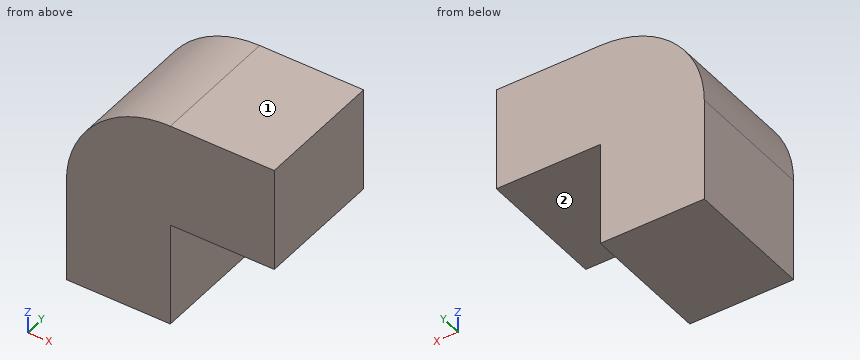
from build123d import *

# Parameters (mm, degrees)
SKETCH_1_W      = 4
SKETCH_1_H      = 5
EXTRUDE_1_DEPTH = 8
SKETCH_2_W      = 4
SKETCH_2_H      = 5
EXTRUDE_2_DEPTH = 4
FILLET_2_R      = 4


with BuildPart() as part:
    # 草图1 → 凸台-拉伸1 (new body)
    with BuildSketch(Plane.XY):
        with Locations((2, -2.5)):
            Rectangle(SKETCH_1_W, SKETCH_1_H)
    extrude(amount=EXTRUDE_1_DEPTH)

    # 草图2 → 凸台-拉伸2 (add)
    with BuildSketch(Plane(origin=(4, 0, 0), x_dir=(0, 0, -1), z_dir=(1, 0, 0))):
        with Locations((-6, -2.5)):
            Rectangle(SKETCH_2_W, SKETCH_2_H)
    extrude(amount=EXTRUDE_2_DEPTH)

    # 圆角2
    fillet_2_edges = [part.edges().sort_by_distance(p)[0] for p in [
        (0, -2.5, 8),
    ]]
    fillet(fillet_2_edges, radius=FILLET_2_R)


solid = part.part
Work out the finished part from the listing and answer in its coordinate system (mm). Face numbers are marked on the shaded views. A direction names the side the tool comes from. Coordinates: 2 decimals unless noted, no trailing zeros. Loops run counter-clockwise (first coordinate to the right, second up) from the corner with the lowest first, then second, coordinate; pieces in that order, holes last. Notation, with made-up numbers: M -34,-7.5 L -25,-7.5 A22 cw -25,24.5 Z; hole C 12,-7 d3. An arc over 180 degrees is marked long. Answer in a Markdown table with one row per item. Add a question column.
1. Find section C-C, the plane x = 4.5. Write down the section's boundary in (y, z), then the cut area to 3 significant figures.
2. Find section B-B, the plane z = 2. Write down the section's boundary in (x, y), then the cut area to 3 significant figures.
3. A flat-ended cylindrical pin translates along its axis: P1, Ø2, axis at x = 5.5, y = -3.5, coming from the -Z side. Find the tip coordinate at first contact, or state that the pin passes through.
4. A tool of negligible diameter and unlimited length cuts with its end or side. For the marked faces 1 and 2, from which of +Z, -Z, +X, -X, +Y, -Y can it reach the whole face along a straight path? Write none if from no direction.
5. Consider L1, parallel to Z at x = 4.25, y = -1; L2, parallel to X at y = -0.85, z = 0.5; L3, parallel to Z at x = 2, y = -3.1. Determine where each line is inside the solid, lowest interval first.
6. Find section A-A, the plane y = -1.65. Write down the section's boundary in (x, z), then the cut area to 3 significant figures.
Reported:
| question | item | result |
|---|---|---|
| 1 | outline | M -5,4 L 0,4 L 0,8 L -5,8 Z |
| 1 | area | 20.0 mm^2 |
| 2 | outline | M 0,-5 L 4,-5 L 4,0 L 0,0 Z |
| 2 | area | 20.0 mm^2 |
| 3 | P1 | stops at z = 4 |
| 4 | face 1 | +Z, +X, -X, +Y, -Y |
| 4 | face 2 | -Z, +X, +Y, -Y |
| 5 | L1 | z = 4 to 8 |
| 5 | L2 | x = 0 to 4 |
| 5 | L3 | z = 0 to 7.46 |
| 6 | outline | M 0,0 L 4,0 L 4,4 L 8,4 L 8,8 L 4,8 A4 ccw 0,4 Z |
| 6 | area | 44.6 mm^2 |
